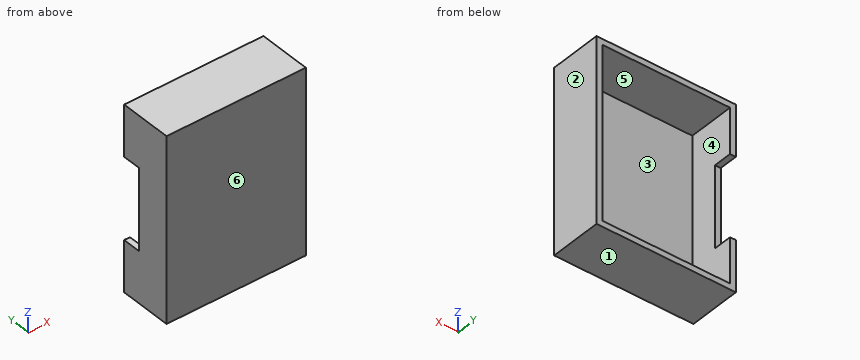
```python
from build123d import *

# Parameters (mm, degrees)
SKETCH1_W           = 120
SKETCH1_H           = 158
SKETCH1_W_2         = 110
SKETCH1_H_2         = 148
BOSS_EXTRUDE1_DEPTH = 40
SKETCH2_W           = 120
SKETCH2_H           = 158
BOSS_EXTRUDE2_DEPTH = 5
SKETCH3_W           = 5
SKETCH3_H           = 70
CUT_EXTRUDE1_DEPTH  = 16


with BuildPart() as part:
    # Sketch1 → Boss-Extrude1 (new body)
    with BuildSketch(Plane(origin=(0, 0, 0), x_dir=(1, 0, 0), z_dir=(0, 1, 0))):
        Rectangle(SKETCH1_W, SKETCH1_H)
        Rectangle(SKETCH1_W_2, SKETCH1_H_2, mode=Mode.SUBTRACT)
    extrude(amount=BOSS_EXTRUDE1_DEPTH)

    # Sketch2 → Boss-Extrude2 (add)
    with BuildSketch(Plane.XZ):
        Rectangle(SKETCH2_W, SKETCH2_H)
    extrude(amount=BOSS_EXTRUDE2_DEPTH)

    # Sketch3 → Cut-Extrude1 (cut)
    with BuildSketch(Plane(origin=(0, 40, 0), x_dir=(1, 0, 0), z_dir=(0, 1, 0))):
        with Locations((-57.5, 0)):
            Rectangle(SKETCH3_W, SKETCH3_H)
    extrude(amount=-CUT_EXTRUDE1_DEPTH, mode=Mode.SUBTRACT)


solid = part.part
```
Can you work these out from the model? Positions are in its coordinate system, mm. Face numbers are marked on the shaded views. A direction names the side the tool comes from. Coordinates: 2 decimals unless noted, no trailing zeros. Loops run counter-clockwise (first coordinate to the right, second up) from the corner with the lowest first, then second, coordinate; pieces in that order, holes last.
Item 1: I'm going to push a flat-ended pin straight in: pin 1 (2.5 mm diameter, centred on x = -57.5, z = -13, fed in from +Y). Where does the tip first touch, or does it pass through?
Answers below:
pin 1: stops at y = 24
Item 2: Suppose I cut it at B-B (z = 12). Please give me the cut outline in (x, y).
Answers below:
outline: (-60, -5) - (60, -5) - (60, 40) - (55, 40) - (55, 0) - (-55, 0) - (-55, 24) - (-60, 24) - close
Item 3: Suppose I cut it at C-C (x = -26). Please give me the cut outline in (y, z).
Answers below:
outline: (-5, -79) - (40, -79) - (40, -74) - (0, -74) - (0, 74) - (40, 74) - (40, 79) - (-5, 79) - close
Item 4: Suppose I cut it at D-D (y = 29). Please give me the cut outline in (x, z), then the cut area to 3 significant figures.
Answers below:
outline: (-60, -79) - (60, -79) - (60, 79) - (-60, 79) - (-60, 35) - (-55, 35) - (-55, 74) - (55, 74) - (55, -74) - (-55, -74) - (-55, -35) - (-60, -35) - close
area: 2,330 mm2
Item 5: Suppose I cut it at A-A (y = 21). Please give me the cut outline in (x, z), then the cut area to 3 significant figures.
Answers below:
outline: (-60, -79) - (60, -79) - (60, 79) - (-60, 79) - close; hole (-55, -74) - (55, -74) - (55, 74) - (-55, 74) - close
area: 2,680 mm2
Item 6: Please list where these lines run through material, in increasing order: L1, parallel to Z at x = 38.5, y = 3.5; L2, parallel to X at y = 13.5, z = 67.5; L3, parallel to Y at x = -42, z = -71.
Answers below:
L1: z = -79 to -74, 74 to 79
L2: x = -60 to -55, 55 to 60
L3: y = -5 to 0
Item 7: If we mould it in two halves opening along Z, with no side actions, what happens to the marked faces 1, 2, 3 and 4? For each: released by +Z, released by -Z, zero draft, split by the parting line, or undercut.
Answers below:
face 1: released by -Z
face 2: zero draft
face 3: undercut
face 4: undercut
Item 8: Which directions (+Z, -Z, +X, -X, +Y, -Y) give clear straight access to the entire face, cutting with the end or side of a thin tool? Please do the marked faces 5 and 6.
Answers below:
face 5: +Y
face 6: +Z, -Z, +X, -X, -Y
